Verification items for the finished model (mm, model axes). A direction names the side the tool comes from. Coordinates: 2 decimals unless noted, no trailing zeros. Write each loop counter-clockwise with the first axis right and the second up, starting at its lowest first coordinate (ties: lowest second). Pieces come first, ordered by that corner, then holes. Notation, with made-up numbers: M -24,-30 L 16,-30 A27 ccw 16,7 Z; hole C -9,-26.5 d8. An arc over 180 degrees is marked long. One line per item, written item: value.
Autodesk Fusion 360 part; units mm, degrees
sketch "Sketch1" plane through (0, 0, 0) normal (0, 1, 0) x (1, 0, 0)
  circle A0 centre (0, 0) radius 13.5
  line L0 (9.0692, -10) -> (9.0692, 10)
  line L1 (9.0692, 10) -> (21.0692, 10)
  line L2 (21.0692, 10) -> (21.0692, -10)
  line L3 (21.0692, -10) -> (9.0692, -10)
  line L4 (9.0692, -10) -> (9.0692, 10)
  dimension "d1" = 27
  dimension "d4" = 20
  dimension "d5" = 12
  dimension "d6" = 20
extrude "Extrude1" add sketch "Sketch1" along normal blind 3
sketch "Sketch2" plane through (0, 3, 0) normal (0, 1, 0) x (-1, 0, 0)
  arc A0 (-9.0692, -10) -> (-9.0692, 10) centre (0, 0) ccw
  line L0 (-9.0692, 10) -> (-21.0692, 10)
  line L1 (-21.0692, 10) -> (-21.0692, -10)
  line L2 (-21.0692, -10) -> (-9.0692, -10)
  circle A1 centre (0, 0) radius 1.5
  dimension "d11" = 3
extrude "Extrude2" cut sketch "Sketch2" against normal blind 7 contours A1
sketch "Sketch3" plane through (0, 3, 0) normal (0, 1, 0) x (-1, 0, 0)
  circle A0 centre (0, 0) radius 1.5
  arc A1 (-9.0692, -10) -> (-9.0692, 10) centre (0, 0) ccw
  line L0 (-9.0692, 10) -> (-21.0692, 10)
  line L1 (-21.0692, 10) -> (-21.0692, -10)
  line L2 (-21.0692, -10) -> (-9.0692, -10)
  line L3 (0, 0) -> (7.2478, -7.2478) construction
  line L4 (0, 0) -> (-7.2478, 7.2478) construction
  line L5 (0, 0) -> (7.2478, 7.2478) construction
  line L6 (0, 0) -> (10.5, 0) construction
  line L7 (0, 0) -> (-7.2478, -7.2478) construction
  line L8 (-7.2478, 7.2478) -> (-6.1872, 8.3085) construction
  line L9 (7.2478, 7.2478) -> (8.3085, 6.1872) construction
  line L10 (7.2478, -7.2478) -> (6.1872, -8.3085) construction
  line L11 (-7.2478, -7.2478) -> (-8.3085, -6.1872) construction
  line L12 (-8.3085, -6.1872) -> (-4.773, -2.6517)
  line L13 (-4.773, -2.6517) -> (-2.6517, -4.773)
  line L14 (-4.773, -2.6517) -> (-1.773, -2.6517) construction
  line L15 (-2.6517, -4.773) -> (-6.1872, -8.3085)
  line L16 (-6.1872, -8.3085) -> (-8.3085, -6.1872)
  line L17 (-6.1872, 8.3085) -> (-8.3085, 6.1872)
  line L18 (-8.3085, 6.1872) -> (-4.773, 2.6517)
  line L19 (-4.773, 2.6517) -> (-2.6517, 4.773)
  line L20 (-4.773, 2.6517) -> (-1.773, 2.6517) construction
  line L21 (-2.6517, 4.773) -> (-6.1872, 8.3085)
  line L22 (8.3085, 6.1872) -> (6.1872, 8.3085)
  line L23 (6.1872, 8.3085) -> (2.6517, 4.773)
  line L24 (6.1872, 8.3085) -> (11.1872, 8.3085) construction
  line L25 (2.6517, 4.773) -> (4.773, 2.6517)
  line L26 (4.773, 2.6517) -> (8.3085, 6.1872)
  line L27 (6.1872, -8.3085) -> (8.3085, -6.1872)
  line L28 (8.3085, -6.1872) -> (4.773, -2.6517)
  line L29 (4.773, -2.6517) -> (2.6517, -4.773)
  line L30 (2.6517, -4.773) -> (6.1872, -8.3085)
  dimension "d15" = 10.25
  dimension "d16" = 10.25
  dimension "d18" = 45
  dimension "d19" = 10.25
  dimension "d20" = 10.25
  dimension "d79" = 1.5
  dimension "d80" = 1.5
  dimension "d81" = 1.5
  dimension "d84" = 1.5
  dimension "d85" = 5
  dimension "d86" = 45
  dimension "d87" = 3
  dimension "d88" = 5
  dimension "d89" = 3
  dimension "d90" = 5
  dimension "d91" = 45
  dimension "d92" = 3
  dimension "d93" = 3
  dimension "d94" = 135
  dimension "d95" = 5
  dimension "d96" = 3
  dimension "d97" = 3
  dimension "d98" = 5
  dimension "d99" = 3
extrude "Extrude12" add sketch "Sketch3" along normal blind 2 contours L12 L13 L15 L16 | L17 L18 L19 L21 | L22 L23 L25 L26 | L27 L28 L29 L30
sketch "Sketch4" plane through (0, 3, 0) normal (0, 1, 0) x (-1, 0, 0)
  circle A0 centre (0, 0) radius 1.5
  arc A1 (-9.0692, -10) -> (-9.0692, 10) centre (0, 0) ccw
  line L0 (-9.0692, 10) -> (-21.0692, 10)
  line L1 (-21.0692, 10) -> (-21.0692, -10)
  line L2 (-21.0692, -10) -> (-9.0692, -10)
  circle A2 centre (0, 0) radius 3.4
  circle A3 centre (0, 0) radius 4.125
  line L3 (-2.6517, 4.773) -> (-4.773, 2.6517)
  line L4 (-4.773, 2.6517) -> (-8.3085, 6.1872)
  line L5 (-8.3085, 6.1872) -> (-6.1872, 8.3085)
  line L6 (-6.1872, 8.3085) -> (-2.6517, 4.773)
  line L7 (4.773, 2.6517) -> (2.6517, 4.773)
  line L8 (2.6517, 4.773) -> (6.1872, 8.3085)
  line L9 (6.1872, 8.3085) -> (8.3085, 6.1872)
  line L10 (8.3085, 6.1872) -> (4.773, 2.6517)
  line L11 (-6.1872, -8.3085) -> (-8.3085, -6.1872)
  line L12 (-8.3085, -6.1872) -> (-4.773, -2.6517)
  line L13 (-4.773, -2.6517) -> (-2.6517, -4.773)
  line L14 (-2.6517, -4.773) -> (-6.1872, -8.3085)
  line L15 (2.6517, -4.773) -> (4.773, -2.6517)
  line L16 (4.773, -2.6517) -> (8.3085, -6.1872)
  line L17 (8.3085, -6.1872) -> (6.1872, -8.3085)
  line L18 (6.1872, -8.3085) -> (2.6517, -4.773)
  dimension "d42" = 6.8
  dimension "d43" = 8.25
extrude "Extrude4" cut sketch "Sketch4" against normal blind 1 contours A3
sketch "Sketch5" plane through (0, 3, 0) normal (0, 1, 0) x (-1, 0, 0)
  arc A0 (-9.0692, -10) -> (-9.0692, 10) centre (0, 0) ccw
  line L0 (-9.0692, 10) -> (-21.0692, 10)
  line L1 (-21.0692, 10) -> (-21.0692, -10)
  line L2 (-21.0692, -10) -> (-9.0692, -10)
  circle A1 centre (0, 0) radius 4.125
  line L3 (-21.0692, -10) -> (-31.0692, -10)
  line L4 (-31.0692, -10) -> (-31.0692, 10)
  line L5 (-31.0692, 10) -> (-21.0692, 10)
  line L6 (-21.0692, 10) -> (-21.0692, -10)
  line L7 (2.6517, -4.773) -> (4.773, -2.6517)
  line L8 (4.773, -2.6517) -> (8.3085, -6.1872)
  line L9 (8.3085, -6.1872) -> (6.1872, -8.3085)
  line L10 (6.1872, -8.3085) -> (2.6517, -4.773)
  line L11 (-6.1872, -8.3085) -> (-8.3085, -6.1872)
  line L12 (-8.3085, -6.1872) -> (-4.773, -2.6517)
  line L13 (-4.773, -2.6517) -> (-2.6517, -4.773)
  line L14 (-2.6517, -4.773) -> (-6.1872, -8.3085)
  line L15 (4.773, 2.6517) -> (2.6517, 4.773)
  line L16 (2.6517, 4.773) -> (6.1872, 8.3085)
  line L17 (6.1872, 8.3085) -> (8.3085, 6.1872)
  line L18 (8.3085, 6.1872) -> (4.773, 2.6517)
  line L19 (-2.6517, 4.773) -> (-4.773, 2.6517)
  line L20 (-4.773, 2.6517) -> (-8.3085, 6.1872)
  line L21 (-8.3085, 6.1872) -> (-6.1872, 8.3085)
  line L22 (-6.1872, 8.3085) -> (-2.6517, 4.773)
  dimension "d46" = 10
  dimension "d47" = 20
extrude "Extrude5" add sketch "Sketch5" along normal blind 16.5 contours L1 L3 L4 L5 L6
sketch "Sketch6" plane through (0, 19.5, 0) normal (0, 1, 0) x (-1, 0, 0)
  line L0 (-21.0692, 10) -> (-31.0692, 10)
  line L1 (-31.0692, 10) -> (-31.0692, -10)
  line L2 (-31.0692, -10) -> (-21.0692, -10)
  line L3 (-21.0692, -10) -> (-21.0692, 10)
  line L4 (-21.0692, 10) -> (-31.0692, 10)
  line L5 (-31.0692, 10) -> (-31.0692, 5)
  line L6 (-31.0692, 5) -> (-21.0692, 5)
  line L7 (-21.0692, 5) -> (-21.0692, 10)
  dimension "d50" = 10
  dimension "d51" = 5
extrude "Extrude6" add sketch "Sketch6" along normal blind 10 contours L0 L1 L3 L4 L5 L6 L7
sketch "Sketch7" plane through (0, 19.5, 0) normal (0, 1, 0) x (-1, 0, 0)
  line L0 (-21.0692, 5) -> (-31.0692, 5)
  line L1 (-31.0692, 5) -> (-31.0692, -10)
  line L2 (-31.0692, -10) -> (-21.0692, -10)
  line L3 (-21.0692, -10) -> (-21.0692, 5)
  line L4 (-21.0692, -10) -> (-21.0692, 10)
  line L5 (-21.0692, 0) -> (-26.0692, 0)
  circle A0 centre (-26.0692, 0) radius 3.4
  dimension "d54" = 5
  dimension "d55" = 6.8
extrude "Extrude7" cut sketch "Sketch7" against normal blind 9 contours A0
sketch "Sketch8" plane through (0, 10.5, 0) normal (0, 1, 0) x (-1, 0, 0)
  circle A0 centre (-26.0692, 0) radius 3.4
  circle A1 centre (-26.0692, 0) radius 1.75
  dimension "d60" = 3.5
sketch "Sketch9" plane through (0, 0, 10) normal (0, 0, 1) x (1, 0, 0)
  line L0 (9.0692, 0) -> (21.0692, 0)
  line L1 (21.0692, 0) -> (21.0692, 3)
  line L2 (21.0692, 3) -> (9.0692, 3)
  line L3 (9.0692, 3) -> (9.0692, 0)
  line L4 (21.0692, 0) -> (27.5513, 6.4821)
  line L5 (21.0692, 0) -> (30.2363, 0) construction
  line L6 (21.0692, 0) -> (21.0692, 3)
  line L7 (31.0692, 3) -> (21.0692, 3)
  line L8 (21.0692, 3) -> (26.0692, 3)
  dimension "d61" = 45
extrude "Extrude8" add sketch "Sketch9" against normal blind 20 contours L1 L4 L6 L7 L8
sketch "Sketch10" plane through (0, 0, 10) normal (0, 0, 1) x (1, 0, 0)
  line L0 (24.0692, 3) -> (31.0692, 3)
  line L1 (31.0692, 3) -> (31.0692, 29.5)
  line L2 (31.0692, 29.5) -> (21.0692, 29.5)
  line L3 (21.0692, 29.5) -> (21.0692, 3)
  line L4 (21.0692, 3) -> (9.0692, 3)
  line L5 (9.0692, 3) -> (9.0692, 0)
  line L6 (9.0692, 0) -> (21.0692, 0)
  line L7 (21.0692, 0) -> (24.0692, 3)
  line L8 (24.0692, 3) -> (32.4914, 11.4222)
  line L9 (24.0692, 3) -> (35.98, 3) construction
  dimension "d64" = 45
extrude "Extrude9" cut sketch "Sketch10" against normal blind 77 contours L0 L1 L8
extrude "Extrude10" cut sketch "Sketch8" against normal blind 20 contours A1
ref_plane "WorkPlane1" through (26.0692, 7.5, 0) normal (0, 1, 0) x (-1, 0, 0)
sketch "Sketch11" plane through (26.0692, 7.5, 0) normal (0, 1, 0) x (1, 0, 0)
  circle A0 centre (0, 0) radius 3
  dimension "d70" = 6
extrude "Extrude11" cut sketch "Sketch11" against normal blind 10
chamfer "Chamfer1" distance 3 angle 45 3 edges at (15.0692, 0, 10) (-13.5, 0, 0) (15.0692, 0, -10)
chamfer "Chamfer2" distance 5 angle 45 1 edges at (21.0692, 3, 0)
chamfer "Chamfer3" distance 3 angle 45 5 edges at (27.5692, 6.5, 10) (31.0692, 19.75, 10) (27.5692, 6.5, -10) (31.0692, 14.75, -10) (31.0692, 10, 0)
fillet "Fillet2" radius 1.35 8 edges at (-2.6517, 4, 4.773) (-4.773, 4, 2.6517) (-4.773, 4, -2.6517) (-2.6517, 4, -4.773) (2.6517, 4, -4.773) (4.773, 4, -2.6517) (4.773, 4, 2.6517) (2.6517, 4, 4.773)
extrude "Extrude13" cut 1 faces at (26.7358, 29.5, 6.6667) along direction (0, -1, 0) blind 1
extrude "Extrude14" cut 1 faces at (24.817, 19.5, -7.7716) along direction (0, -1, 0) blind 1
extrude "Extrude15" cut 1 faces at (23.2318, 10.5, -0.1689) along direction (0, -1, 0) blind 1
equation "d5 = KneeSeparation"
equation "d7 = BottomThickness"
equation "BottomThickness = 3 mm"
equation "KneeSeparation = 12 mm"
equation "d11 = ServoScrewHole"
equation "ScrewHole = 3.0 mm"
equation "HornFit = 1.35 mm"
equation "d54 = HolePosX"
equation "d55 = HoleSize"
equation "HolePosX = 5 mm"
equation "HoleSize = 6.8 mm"
equation "d60 = SpacerScrewHole"
equation "d70 = HoleFit"
equation "HoleFit = 6 mm"
equation "ChamferStrength = 5 mm"
equation "Chamfer3 = 3 mm"
equation "d76 = Chamfer3"
equation "d77 = ChamferStrength"
equation "d78 = Chamfer3"
equation "FilletFIT = 1.35 mm"
equation "d103 = FilletFIT"
equation "HoleDepth = 9 mm"
equation "ServoScrewHole = 3 mm"
equation "SpacerScrewHole = 3.5 mm"
Item 1: Cross-section at C-C, the plane y = 13.75. Enter the section's corners in (x, z).
The answers:
outline: M 21.07,-10 L 28.07,-10 L 31.07,-7 L 31.07,7 L 28.07,10 L 21.07,10 Z; hole C 26.07,0 d6.8
Item 2: Go/stop test with flat-tipped pins: P1, Ø3.5, axis at x = 0.5, z = -0.5, coming from the +Y side; P2, Ø8, axis at x = 26.07, z = 0, coming from the +Y side; P3, Ø6, axis at y = 13.5, z = 6, coming from the -X side; P4, Ø6, axis at y = 22.5, z = -3.5, coming from the -X side. Record where each tip stops, or that it passes through.
The answers:
P1: stops at y = 3
P2: stops at y = 18.5
P3: stops at x = 21.07
P4: passes through
Item 3: Access from +Z, -Z, +X, -X, +Y, -Y to the whole of each face (thin tool, end or side, straight path). Record for faces 1 (the face through (26, 23, 5)), 2 (the face through (4.88, 3.99, -7)), 3 (the face through (-7.233, 3.986, -7.263)), 4 (the face through (15, 2, -9)), 5 (the face through (7.036, 3.986, -4.915)).
The answers:
face 1: -Z, +X, -X, +Y
face 2: -Z, +Y
face 3: -Z, -X, +Y
face 4: -Z, +X, -Y
face 5: +Y
Item 4: Scan lines: line 1 (Z direction, x = 25.5, y = 26.75); line 2 (X direction, y = 25.25, z = 7); line 3 (X direction, y = 10, z = -0.5). Record each from-to range of solid material in increasing order.
The answers:
line 1: z = 5 to 10
line 2: x = 21.07 to 31.07
line 3: x = 21.07 to 22.71, 29.43 to 29.83
Item 5: Cross-section at A-A, the plane z = 0. Give the number of separate pieces and of enclosed holes in the cut face, and give its area (3 significant figures).
The answers:
separate pieces: 3
enclosed holes: 0
area: 150 mm²
Item 6: Draft check along Z on faces 6 (the face through (21.069, 16, 2)), 7 (the face through (28, 9.5, 1)), 8 (the face through (24.02, 5.04, -8.48)). Enter one of: released by +Z, released by -Z, zero draft, split by the parting line, or undercut.
The answers:
face 6: zero draft
face 7: undercut
face 8: released by -Z
